Model file for the job. Use its own axes, mm. A direction names the side the tool comes from. Give positions to 0.01 mm unless a question says otherwise; leave off trailing zeros. Loops run counter-clockwise (first coordinate to the right, second up) from the corner with the lowest first, then second, coordinate; pieces in that order, holes last. Notation, with made-up numbers: M 66.5,-25 L 120.5,-25 A20 ccw 120.5,10 Z; hole C 47,16 d9. An arc over 180 degrees is marked long. Answer in a Markdown table with one row per item.
```python
from build123d import *

# Parameters (mm, degrees)
SKETCH1_R           = 5.9
SKETCH1_W           = 6.4
SKETCH1_H           = 6.4
BOSS_EXTRUDE1_DEPTH = 5.5
BOSS_EXTRUDE2_START = 2
SKETCH1_3_R         = 8
SKETCH1_3_R_2       = 5.9
SKETCH1_3_W         = 6.4
SKETCH1_3_H         = 6.4
BOSS_EXTRUDE2_DEPTH = 2
FILLET1_R           = 0.5
CUT_EXTRUDE1_DEPTH  = 0.5


with BuildPart() as part:
    # Sketch1 → Boss-Extrude1 (new body)
    with BuildSketch(Plane.XY):
        Circle(SKETCH1_R)
        Rectangle(SKETCH1_W, SKETCH1_H, mode=Mode.SUBTRACT)
    extrude(amount=-BOSS_EXTRUDE1_DEPTH)

    # Sketch1_3 → Boss-Extrude2 (add)
    # profile 1 of 2: a face of its own
    with BuildSketch(Plane.XY.offset(BOSS_EXTRUDE2_START)):
        Circle(SKETCH1_3_R)
        Circle(SKETCH1_3_R_2, mode=Mode.SUBTRACT)
    # profile 2 of 2: a face of its own
    with BuildSketch(Plane.XY.offset(BOSS_EXTRUDE2_START)):
        Circle(SKETCH1_3_R_2)
        Rectangle(SKETCH1_3_W, SKETCH1_3_H, mode=Mode.SUBTRACT)
    extrude(amount=-BOSS_EXTRUDE2_DEPTH)

    # Fillet1
    fillet1_edges = [part.edges().sort_by_distance(p)[0] for p in [
        (-8, 0, 0),
        (-5.9, 0, -5.5),
    ]]
    fillet(fillet1_edges, radius=FILLET1_R)

    # Sketch2 → Cut-Extrude1 (cut)
    with BuildSketch(Plane.XY.offset(2)):
        Polygon((-0.475804426, 7.144860485), (0.171330991, 7.144860485), (0.171330991, 3.644860485), (-0.142771573, 3.644860485), (-0.142771573, 6.785886126), (-0.681233112, 6.785886126), align=None)
    extrude(amount=-CUT_EXTRUDE1_DEPTH, mode=Mode.SUBTRACT)


solid = part.part
```
Q1. Drop flat-ended pins along their axis: pin 1 (1 mm diameter, centred on x = -5.5, z = -3, fed in from +Y); pin 2 (1.9 mm diameter, centred on x = 1, z = -3, fed in from -Y); pin 3 (0.6 mm diameter, centred on y = 6, z = 1.5, fed in from -X); pin 4 (0.9 mm diameter, centred on x = 0, y = 4.5, fed in from +Z). Give the stop position or say it passes through.
Reported:
| item | result |
|---|---|
| pin 1 | y = 3.13 |
| pin 2 | y = -5.9 |
| pin 3 | x = -5.61 |
| pin 4 | z = 2 |
Q2. Probe probe 1 along Z at (x, y) = (-5.75, 4); probe 2 along X at (y, z) = (-2.25, -0.25); probe 3 along Y at (x, z) = (-3, -4). List the from-to ranges inside material, lowest first.
Reported:
| item | result |
|---|---|
| probe 1 | 0 to 2 |
| probe 2 | -5.45 to -3.2, 3.2 to 5.45 |
| probe 3 | -5.08 to -3.2, 3.2 to 5.08 |
Q3. Saw through at B-B (z = -2). Give the cut face in (x, y), and give its area (3 significant figures).
Reported:
| item | result |
|---|---|
| outline | C 0,0 d11.8; hole M -3.2,-3.2 L 3.2,-3.2 L 3.2,3.2 L -3.2,3.2 Z |
| area | 68.4 mm² |
Q4. Saw through at A-A (y = 0). Give the cut face in (x, z), and give its area (3 significant figures).
Reported:
| item | result |
|---|---|
| outline | M -8,0.5 A0.5 ccw -7.5,0 L -5.9,0 L -5.9,-5 A0.5 ccw -5.4,-5.5 L -3.2,-5.5 L -3.2,2 L -8,2 Z; M 3.2,-5.5 L 5.4,-5.5 A0.5 ccw 5.9,-5 L 5.9,0 L 7.5,0 A0.5 ccw 8,0.5 L 8,2 L 3.2,2 Z |
| area | 48.7 mm² |
Q5. Mould opens along X. For faces 4 (the face through (-5.894, 0.259, -2.465)), 5 (the face through (-0.1, -3.4, 2)), 6 (the face through (-3.2, 0, -2)) say: released by +X, released by -X, zero draft, split by the parting line, or undercut.
Reported:
| item | result |
|---|---|
| face 4 | split by the parting line |
| face 5 | zero draft |
| face 6 | undercut |
Q6. 3-axis set-ups, long thin cutter, end or side, ignore diameter. For faces 1 (the face through (0, -4, -5.5)), 2 (the face through (-6, -2, 0)), 3 (the face through (0, -3.2, -2)): which of +Z, -Z, +X, -X, +Y, -Y reach the whole face in a straight line?
Reported:
| item | result |
|---|---|
| face 1 | -Z, +X, -X, +Y, -Y |
| face 2 | -Z |
| face 3 | +Z, -Z |
